from build123d import *

# Parameters (mm, degrees)
SKETCH1_R           = 1.75
BOSS_EXTRUDE3_DEPTH = 3
SKETCH4_W           = 38.009499712
SKETCH4_H           = 2.5
CUT_EXTRUDE7_DEPTH  = 29.268853886
SKETCH7_W           = 36
SKETCH7_H           = 1
CUT_EXTRUDE8_DEPTH  = 47.877632193
SKETCH9_W           = 39.982004405
SKETCH9_H           = 3.901650926
SKETCH9_W_2         = 38.509499712
SKETCH9_H_2         = 2.8
SKETCH9_W_3         = 37.982004405
SKETCH9_H_3         = 0.55
CUT_EXTRUDE9_DEPTH  = 10
SKETCH10_W          = 40
SKETCH10_H          = 4
SKETCH10_W_2        = 39.982004405
SKETCH10_H_2        = 3.901650926
CUT_EXTRUDE11_DEPTH = 29.180278565
SKETCH11_W          = 20
SKETCH11_H          = 3.116121774
CUT_EXTRUDE12_DEPTH = 10
SKETCH12_W          = 2
SKETCH12_H          = 8.5
CUT_EXTRUDE15_DEPTH = 10


with BuildPart() as part:
    # Sketch1 → Boss-Extrude3 (new body)
    # profile 1 of 2: a face of its own
    with BuildSketch(Plane(origin=(0, 0, 0), x_dir=(1, 0, 0), z_dir=(0, 1, 0))):
        Polygon((-21.59, 18), (-21.59, 0), (0, 0), (21.59, 0), (21.59, 18), (18.04585781, 18), (10.04585781, 18), (10.04585781, 12.616121774), (-9.95414219, 12.616121774), (-9.95414219, 18), (-17.95414219, 18), align=None)
        with Locations(Location((-15, 15, 0), (0, 0, 270))):
            Circle(SKETCH1_R, mode=Mode.SUBTRACT)
        Polygon((18.504745017, 6.25), (0, 6.25), (-18.5, 6.25), (-19.004539265, 6.25), (-19.004539265, 8.75), (-18.5, 8.75), (0.002372509, 8.75), (18.504745017, 8.75), (19.004960447, 8.75), (19.004960447, 6.25), align=None, mode=Mode.SUBTRACT)
        with Locations(Location((15, 15, 0), (0, 0, 270))):
            Circle(SKETCH1_R, mode=Mode.SUBTRACT)
    # profile 2 of 2: a face of its own
    with BuildSketch(Plane(origin=(0, 0, 0), x_dir=(1, 0, 0), z_dir=(0, 1, 0))):
        Polygon((0, 0), (-21.59, 0), (-21.59, -18), (-17.95414219, -18), (-9.95414219, -18), (-9.95414219, -12.616121774), (10.04585781, -12.616121774), (10.04585781, -18), (18.04585781, -18), (21.59, -18), (21.59, 0), align=None)
        with Locations(Location((-15, -15, 0), (0, 0, 270))):
            Circle(SKETCH1_R, mode=Mode.SUBTRACT)
        with Locations(Location((15, -15, 0), (0, 0, 270))):
            Circle(SKETCH1_R, mode=Mode.SUBTRACT)
        Polygon((18.504745017, -6.25), (19.004960447, -6.25), (19.004960447, -8.75), (18.504745017, -8.75), (-18.5, -8.75), (-19.004539265, -8.75), (-19.004539265, -6.25), (-18.5, -6.25), align=None, mode=Mode.SUBTRACT)
    extrude(amount=BOSS_EXTRUDE3_DEPTH)

    # Sketch4 → Cut-Extrude7 (cut, through all)
    # profile 1 of 3: a face of its own
    with BuildSketch(Plane(origin=(0, 3, 0), x_dir=(1, 0, 0), z_dir=(0, 1, 0))):
        Polygon((19.004960447, 6.1), (19.254960447, 6.1), (19.254960447, 8.882786661), (19.254960447, 8.9), (19.004960447, 8.9), (-19.004539265, 8.9), (-19.254539265, 8.9), (-19.254539265, 6.1), (-19.004539265, 6.1), align=None)
        with Locations((0.000210591, 7.5)):
            Rectangle(SKETCH4_W, SKETCH4_H, mode=Mode.SUBTRACT)
    # profile 2 of 3: a face of its own
    with BuildSketch(Plane(origin=(0, 3, 0), x_dir=(1, 0, 0), z_dir=(0, 1, 0))):
        with Locations((0.000210591, 7.5)):
            Rectangle(SKETCH4_W, SKETCH4_H)
    # profile 3 of 3: a face of its own
    with BuildSketch(Plane(origin=(0, 3, 0), x_dir=(1, 0, 0), z_dir=(0, 1, 0))):
        Polygon((-19.254539265, -6.1), (-19.254539265, -8.9), (-19.004539265, -8.9), (19.004960447, -8.9), (19.254960447, -8.9), (19.254960447, -6.1), (19.004960447, -6.1), (-19.004539265, -6.1), align=None)
        with Locations((0.000210591, -7.5)):
            Rectangle(SKETCH4_W, SKETCH4_H, mode=Mode.SUBTRACT)
    extrude(amount=-CUT_EXTRUDE7_DEPTH, mode=Mode.SUBTRACT)

    # Sketch7 → Cut-Extrude8 (cut, through all)
    with BuildSketch(Plane(origin=(21.59, 0, 0), x_dir=(0, 0, -1), z_dir=(1, 0, 0))):
        with Locations((0, 0.5)):
            Rectangle(SKETCH7_W, SKETCH7_H)
    extrude(amount=-CUT_EXTRUDE8_DEPTH, mode=Mode.SUBTRACT)

    # Sketch9 → Cut-Extrude9 (cut)
    # profile 1 of 4: a face of its own
    with BuildSketch(Plane(origin=(0, 3, 0), x_dir=(1, 0, 0), z_dir=(0, 1, 0))):
        with Locations((0.000210592, 7.5)):
            Rectangle(SKETCH9_W, SKETCH9_H)
        with Locations((0.000210591, 7.5)):
            Rectangle(SKETCH9_W_2, SKETCH9_H_2, mode=Mode.SUBTRACT)
    # profile 2 of 4: a face of its own
    with BuildSketch(Plane(origin=(0, 3, 0), x_dir=(1, 0, 0), z_dir=(0, 1, 0))):
        with Locations((0.000210592, -7.5)):
            Rectangle(SKETCH9_W, SKETCH9_H)
        Polygon((-19.254539265, -8.9), (-19.254539265, -6.1), (-18.990791611, -6.1), (-18.990791611, -5.55), (18.991212794, -5.55), (18.991212794, -6.1), (19.254960447, -6.1), (19.254960447, -8.9), (18.991212794, -8.9), (18.991212794, -9.45), (-18.990791611, -9.45), (-18.990791611, -8.9), align=None, mode=Mode.SUBTRACT)
    # profile 3 of 4: a face of its own
    with BuildSketch(Plane(origin=(0, 3, 0), x_dir=(1, 0, 0), z_dir=(0, 1, 0))):
        with Locations((0.000210592, -5.825)):
            Rectangle(SKETCH9_W_3, SKETCH9_H_3)
    # profile 4 of 4: a face of its own
    with BuildSketch(Plane(origin=(0, 3, 0), x_dir=(1, 0, 0), z_dir=(0, 1, 0))):
        with Locations((0.000210592, -9.175)):
            Rectangle(SKETCH9_W_3, SKETCH9_H_3)
    extrude(amount=-CUT_EXTRUDE9_DEPTH, mode=Mode.SUBTRACT)

    # Sketch10 → Cut-Extrude11 (cut, through all)
    # profile 1 of 3: a face of its own
    with BuildSketch(Plane(origin=(0, 3, 0), x_dir=(1, 0, 0), z_dir=(0, 1, 0))):
        with Locations((0.000210591, -7.5)):
            Rectangle(SKETCH10_W, SKETCH10_H)
        with Locations((0.000210592, -7.5)):
            Rectangle(SKETCH10_W_2, SKETCH10_H_2, mode=Mode.SUBTRACT)
    # profile 2 of 3: a face of its own
    with BuildSketch(Plane(origin=(0, 3, 0), x_dir=(1, 0, 0), z_dir=(0, 1, 0))):
        with Locations((0.000210591, 7.5)):
            Rectangle(SKETCH10_W, SKETCH10_H)
        with Locations((0.000210592, 7.5)):
            Rectangle(SKETCH10_W_2, SKETCH10_H_2, mode=Mode.SUBTRACT)
    # profile 3 of 3: a face of its own
    with BuildSketch(Plane(origin=(0, 3, 0), x_dir=(1, 0, 0), z_dir=(0, 1, 0))):
        with Locations((0.000210592, 7.5)):
            Rectangle(SKETCH10_W_2, SKETCH10_H_2)
    extrude(amount=-CUT_EXTRUDE11_DEPTH, mode=Mode.SUBTRACT)

    # Sketch11 → Cut-Extrude12 (cut)
    with BuildSketch(Plane(origin=(0, 3, 0), x_dir=(1, 0, 0), z_dir=(0, 1, 0))):
        with Locations((0.04585781, -11.058060887)):
            Rectangle(SKETCH11_W, SKETCH11_H)
        with Locations((0.04585781, 11.058060887)):
            Rectangle(SKETCH11_W, SKETCH11_H)
    extrude(amount=-CUT_EXTRUDE12_DEPTH, mode=Mode.SUBTRACT)

    # Sketch12 → Cut-Extrude15 (cut)
    with BuildSketch(Plane(origin=(0, 3, 0), x_dir=(1, 0, 0), z_dir=(0, 1, 0))):
        with Locations((-10.95414219, -13.75)):
            Rectangle(SKETCH12_W, SKETCH12_H)
        with Locations((-10.95414219, 13.75)):
            Rectangle(SKETCH12_W, SKETCH12_H)
        with Locations((11.04585781, 13.75)):
            Rectangle(SKETCH12_W, SKETCH12_H)
        Polygon((10.04585781, -9.65592739), (10.04585781, -18), (12.04585781, -18), (12.04585781, -9.65592739), (12.04585781, -9.5), (10.04585781, -9.5), align=None)
    extrude(amount=-CUT_EXTRUDE15_DEPTH, mode=Mode.SUBTRACT)


solid = part.part
Design review of the part built by this model. Coordinates are the model's own, in mm. A direction names the side the tool comes from. Round coordinates to 2 decimals unless told otherwise and drop trailing zeros. Write each loop counter-clockwise with the first axis right and the second up, starting at its lowest first coordinate (ties: lowest second). Pieces come first, ordered by that corner, then holes. Notation, with made-up numbers: (85.5, 6) - (124.5, 6) arc R25 ccw to (124.5, 28) - close; hole circle Ø8 at (81.5, 88.25). An arc over 180 degrees is marked (long way). Return JSON: item names as keys, results as strings. Group by question number.
Item 1: Insertion check: P1, Ø3, axis at x = 15, z = -15, coming from the +Y side; P2, Ø1, axis at x = -1, y = 3, coming from the +Z side; P3, Ø4.5, axis at x = -15, z = -15, coming from the -Y side. Each pin has a flat end and moves straight along its axis. Give the tip position at first contact, or say it passes through.
Item 2: For probe 1 along X at (y, z) = (1.6, 15); probe 2 along Z at (x, y) = (-15, 2.5); probe 3 along Z at (x, y) = (-12.5, 1.35), list the stretches that pass through material, from the lowest coordinate up. Write a range as [from, to].
Item 3: We need section A-A on z = -15. Write out the cut boundary in (x, y).
Item 4: We need section C-C on y = 1.95. Write out the cut boundary in (x, z).
Item 5: The part is to be moulded in two halves that separate along Z. For faces 6 (the face through (-21.59, 2, 0)), 7 (the face through (-17, 2, 18)), 8 (the face through (20, 2, 8)), say which applies: pulls with the +Z half, pulls with the -Z half, needs draft (parallel to the pull), parting line crosses it, or undercut.
Item 6: We need section B-B on x = 19. Write out the cut boundary in (y, z), and give its area (3 significant figures).
Item 7: We need section D-D on z = 10. Write out the cut boundary in (x, y), and give its area (3 significant figures).
Item 8: Machinability: for faces 1 (the face through (-11.954, 2, 14)), 2 (the face through (17, 2, 18)), 3 (the face through (21.59, 2, 0)), 4 (the face through (12.046, 2, -14)), 5 (the face through (-20, 2, -7)), which of the approach directions +Z, -Z, +X, -X, +Y, -Y give a long, thin tool a straight path to every point of the face, cutting with its end or side? Answer none if there is none.
Model answer:
{
 "1": {"P1": "passes through", "P2": "stops at z = 5.5", "P3": "stops at y = 1"},
 "2": {"probe 1": "x = [-21.59, -16.75], [-13.25, -11.95], [12.05, 13.25], [16.75, 21.59]", "probe 2": "z = [-18, -16.75], [-13.25, -9.5], [-5.5, 5.5], [9.5, 13.25], [16.75, 18]", "probe 3": "z = [-18, -9.5], [-5.5, 5.5], [9.5, 18]"},
 "3": {"outline": "(-21.59, 1) - (-16.75, 1) - (-16.75, 3) - (-21.59, 3) - close; (-13.25, 1) - (-11.95, 1) - (-11.95, 3) - (-13.25, 3) - close; (12.05, 1) - (13.25, 1) - (13.25, 3) - (12.05, 3) - close; (16.75, 1) - (21.59, 1) - (21.59, 3) - (16.75, 3) - close"},
 "4": {"outline": "(-21.59, -18) - (-11.95, -18) - (-11.95, -9.5) - (-20, -9.5) - (-20, -5.5) - (20, -5.5) - (20, -9.5) - (12.05, -9.5) - (12.05, -18) - (21.59, -18) - (21.59, 18) - (12.05, 18) - (12.05, 9.5) - (20, 9.5) - (20, 5.5) - (-20, 5.5) - (-20, 9.5) - (-11.95, 9.5) - (-11.95, 18) - (-21.59, 18) - close; hole circle Ø3.5 at (-15, -15); hole circle Ø3.5 at (-15, 15); hole circle Ø3.5 at (15, -15); hole circle Ø3.5 at (15, 15)"},
 "5": {"face 6": "needs draft", "face 7": "pulls with the +Z half", "face 8": "undercut"},
 "6": {"outline": "(1, -18) - (3, -18) - (3, -9.5) - (1, -9.5) - close; (1, -5.5) - (3, -5.5) - (3, 5.5) - (1, 5.5) - close; (1, 9.5) - (3, 9.5) - (3, 18) - (1, 18) - close", "area": "56.0 mm²"},
 "7": {"outline": "(-21.59, 1) - (-11.95, 1) - (-11.95, 3) - (-21.59, 3) - close; (12.05, 1) - (21.59, 1) - (21.59, 3) - (12.05, 3) - close", "area": "38.4 mm²"},
 "8": {"face 1": "+Z, +Y, -Y", "face 2": "+Z, +X, -X, +Y, -Y", "face 3": "+Z, -Z, +X, +Y, -Y", "face 4": "-Z, +Y, -Y", "face 5": "+Y, -Y"}
}
